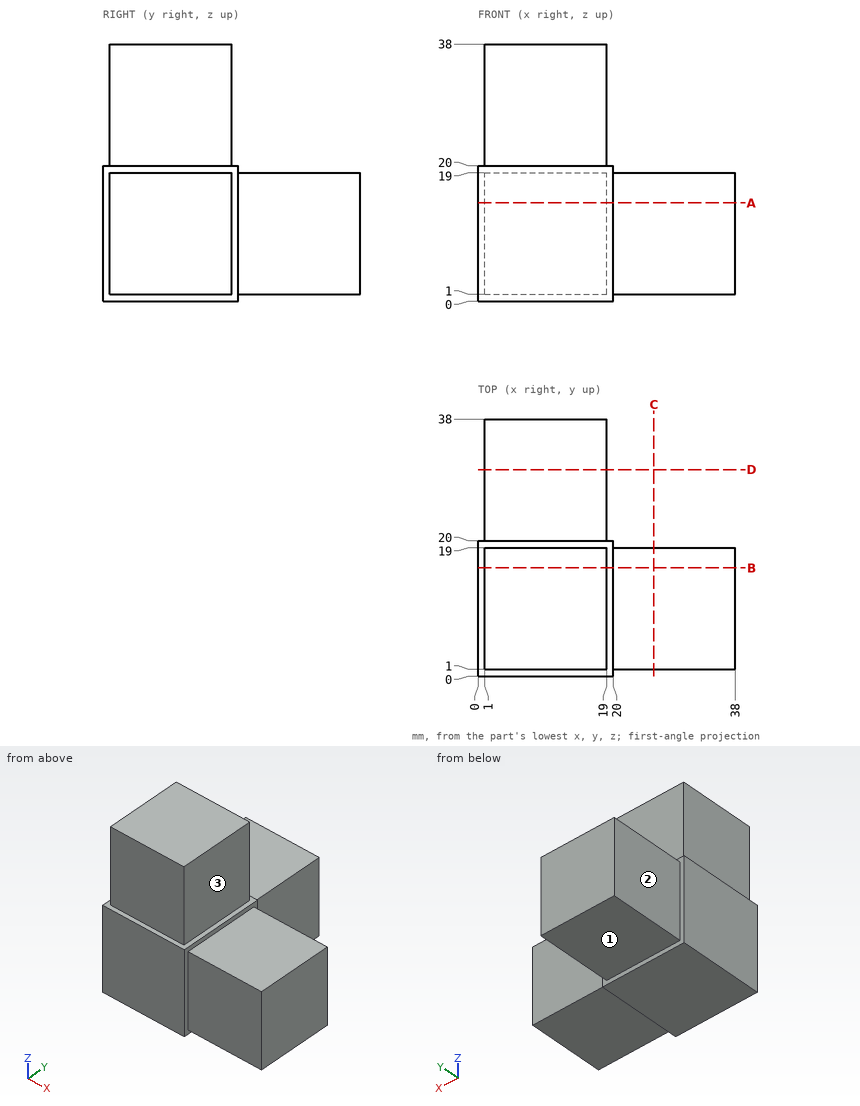
Here's the drawing with two shaded views (mm, measured from the low corner). I have some questions. A direction names the side the tool comes from. Round coordinates to 2 decimals unless told otherwise and drop trailing zeros. Write each loop counter-clockwise with the first axis right and the second up, starting at its lowest first coordinate (ties: lowest second). Pieces come first, ordered by that corner, then holes.
(1) Suppose I cut it at C-C on x = 26. Write out the boundary of the cut face in (y, z), and give its area (3 significant figures).
Findings below:
outline: (1, 1) - (19, 1) - (19, 19) - (1, 19) - close
area: 324 mm2
(2) Suppose I cut it at A-A on z = 14.5. Write out the boundary of the cut face in (x, y), and give its area (3 significant figures).
Findings below:
outline: (0, 0) - (20, 0) - (20, 1) - (38, 1) - (38, 19) - (20, 19) - (20, 20) - (19, 20) - (19, 38) - (1, 38) - (1, 20) - (0, 20) - close
area: 1,050 mm2
(3) For pin 1 (10 mm diameter, centred on x = 24.5, z = 20.5, fed in from +Y); pin 2 (14.5 mm diameter, centred on x = 10.5, z = 30.5, fed in from +Y); pin 3 (14.5 mm diameter, centred on x = 12.5, z = 32.5, fed in from -Y), each with a flat end and sliding along its axis, tell me the tip position at first contact or that it passes through.
Findings below:
pin 1: stops at y = 20
pin 2: stops at y = 19
pin 3: stops at y = 1
(4) Which directions (+Z, -Z, +X, -X, +Y, -Y) give clear straight access to the entire face, cutting with the end or side of a thin tool? Please do the marked faces 1, 2 and 3.
Findings below:
face 1: -Z, +X, -X, +Y
face 2: +Z, -Z, -X, +Y
face 3: +Z, +X, +Y, -Y
(5) If I drill on probe 1 along X at (y, z) = (23, 14); probe 2 along X at (y, z) = (19.5, 9), over which ranges is the centre line in solid material (lowest first)?
Findings below:
probe 1: x = 1 to 19
probe 2: x = 0 to 20
